The model under review builds one solid part; all positions refer to its coordinate system, in mm. Face numbers are marked on the shaded views. A direction names the side the tool comes from. Give positions to 0.01 mm unless a question says otherwise; leave off trailing zeros. Order: outer loops, then holes, each group sorted by start corner. A loop starts at its lowest first (then second) coordinate and runs counter-clockwise, first axis right, second up. Notation, with made-up numbers: (64.5, 30.25) - (79.5, 30.25) arc R31 cw to (79.5, 66.25) - close; hole circle Ø7 at (-38, -29.75). An arc over 180 degrees is marked (long way). Use CSV: the item, a comma, the result in double quotes.
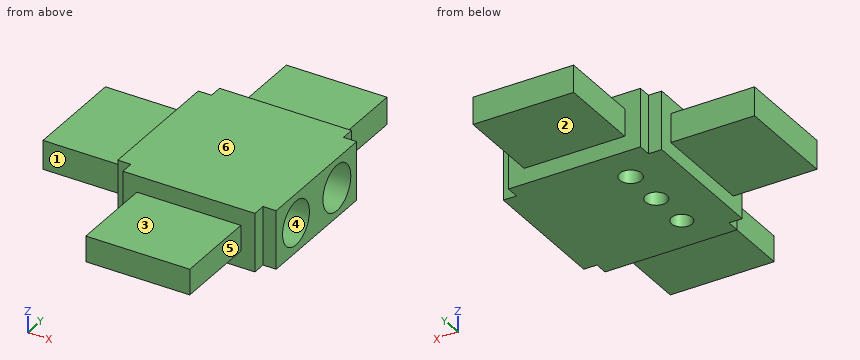
```python
from build123d import *

# Parameters (mm, degrees)
F0_W      = 20
F0_H      = 2
F0_W_2    = 2
F0_H_2    = 20
F1_DEPTH  = 4.445
F2_W      = 15.5
F2_H      = 4.39
F3_DEPTH  = 12.7
F4_W      = 15.75
F4_H      = 3.9
F5_DEPTH  = 12.7
F6_W      = 15.25
F6_H      = 4.14
F7_DEPTH  = 12.7
F8_R      = 3.33175
F8_R_2    = 3.45675
F9_DEPTH  = 7.62
F10_R     = 1.6625
F10_R_2   = 1.625
F10_R_3   = 1.5625
F11_DEPTH = 5.08


with BuildPart() as f1:
    # F0 (on Top) → F1 (new body, symmetric)
    with BuildSketch(Plane.XY):
        with Locations((0, 11)):
            Rectangle(F0_W, F0_H)
        with Locations((11, 0)):
            Rectangle(F0_W_2, F0_H_2)
        Rectangle(F0_W, F0_H_2)
        with Locations((-11, 0)):
            Rectangle(F0_W_2, F0_H_2)
        with Locations((0, -11)):
            Rectangle(F0_W, F0_H)
    extrude(amount=F1_DEPTH, both=True)

    # F2 (on face) → F3 (join)
    with BuildSketch(Plane(origin=(-12, 0, 0), x_dir=(0, -1, 0), z_dir=(-1, 0, 0))):
        Rectangle(F2_W, F2_H)
    extrude(amount=F3_DEPTH)

    # F4 (on face) → F5 (join)
    with BuildSketch(Plane.XZ.offset(12)):
        Rectangle(F4_W, F4_H)
    extrude(amount=F5_DEPTH)

    # F6 (on face) → F7 (join)
    with BuildSketch(Plane(origin=(0, 12, 0), x_dir=(-1, 0, 0), z_dir=(0, 1, 0))):
        Rectangle(F6_W, F6_H)
    extrude(amount=F7_DEPTH)

    # F8 (on face) → F9 (cut)
    with BuildSketch(Plane.YZ.offset(12)):
        with Locations((-5.08, 0)):
            Circle(F8_R)
        with Locations((5.08, 0)):
            Circle(F8_R_2)
    extrude(amount=-F9_DEPTH, mode=Mode.SUBTRACT)

    # F10 (on face) → F11 (cut)
    with BuildSketch(Plane(origin=(0, 0, -4.445), x_dir=(1, 0, 0), z_dir=(0, 0, -1))):
        with Locations((-5.08, -6.35)):
            Circle(F10_R)
        with Locations((-5.08, 0)):
            Circle(F10_R_2)
        with Locations((-5.08, 6.35)):
            Circle(F10_R_3)
    extrude(amount=-F11_DEPTH, mode=Mode.SUBTRACT)


solid = f1.part
```
Item 1: Clearance check with flat-ended pins moving along their axes: pin 1 (1 mm diameter, centred on y = 4.5, z = 1.5, fed in from +X); pin 2 (1.6 mm diameter, centred on y = -10.5, z = -1.5, fed in from -X); pin 3 (2 mm diameter, centred on x = -10.5, z = -0.5, fed in from -Y). State where each tip first meets the part, or that it passes through.
Results list:
pin 1,"stops at x = 4.38"
pin 2,"stops at x = -12"
pin 3,"stops at y = -12"
Item 2: Take a section at B-B, the plane y = 0. Give the boundary of the cut face in (x, z) (3 decimals).
Results list:
outline,"(-24.7, -2.195) - (-12, -2.195) - (-12, -4.445) - (-6.705, -4.445) - (-6.705, 0.635) - (-3.455, 0.635) - (-3.455, -4.445) - (12, -4.445) - (12, 4.445) - (-12, 4.445) - (-12, 2.195) - (-24.7, 2.195) - close"
Item 3: Take a section at D-D, the plane x = 3. Give the boundary of the cut face in (y, z) (3 decimals).
Results list:
outline,"(-24.7, -1.95) - (-12, -1.95) - (-12, -4.445) - (12, -4.445) - (12, -2.07) - (24.7, -2.07) - (24.7, 2.07) - (12, 2.07) - (12, 4.445) - (-12, 4.445) - (-12, 1.95) - (-24.7, 1.95) - close"
Item 4: Take a section at C-C, the plane z = 0. State how many separate pieces and enclosed holes the cut face has, and give its area (3 significant figures).
Results list:
separate pieces,"1"
enclosed holes,"3"
area,"1,020 mm2"
Item 5: Wall thickness on L1, parallel to Y at x = -5.08, z = -1.4 (1 decimal); L2, parallel to Z at x = 6.25, y = -5.08 (3 decimals); L3, parallel to Z at x = 6.25, y = 5.08 (3 decimals): over which ranges is each line inside the solid? List them lowest first.
Results list:
L1,"y = -24.7 to -7.9, -4.8 to -1.6, 1.6 to 4.7, 8 to 24.7"
L2,"z = -4.445 to -3.332, 3.332 to 4.445"
L3,"z = -4.445 to -3.457, 3.457 to 4.445"
Item 6: Mouldability with a two-part tool opening along Z and no side actions: class the marked faces 4, 5 and 6 as pulls with the +Z half, pulls with the -Z half, needs draft (parallel to the pull), parting line crosses it, or undercut.
Results list:
face 4,"undercut"
face 5,"needs draft"
face 6,"pulls with the +Z half"
Item 7: Tool access review of the marked faces 1, 2 and 3: name each direction out of +Z, -Z, +X, -X, +Y, -Y from which nothing blocks a thin tool from reaching the whole face with its end or side.
Results list:
face 1,"+Z, -Z, -X, -Y"
face 2,"-Z, +X, -X, +Y"
face 3,"+Z, +X, -X, -Y"
